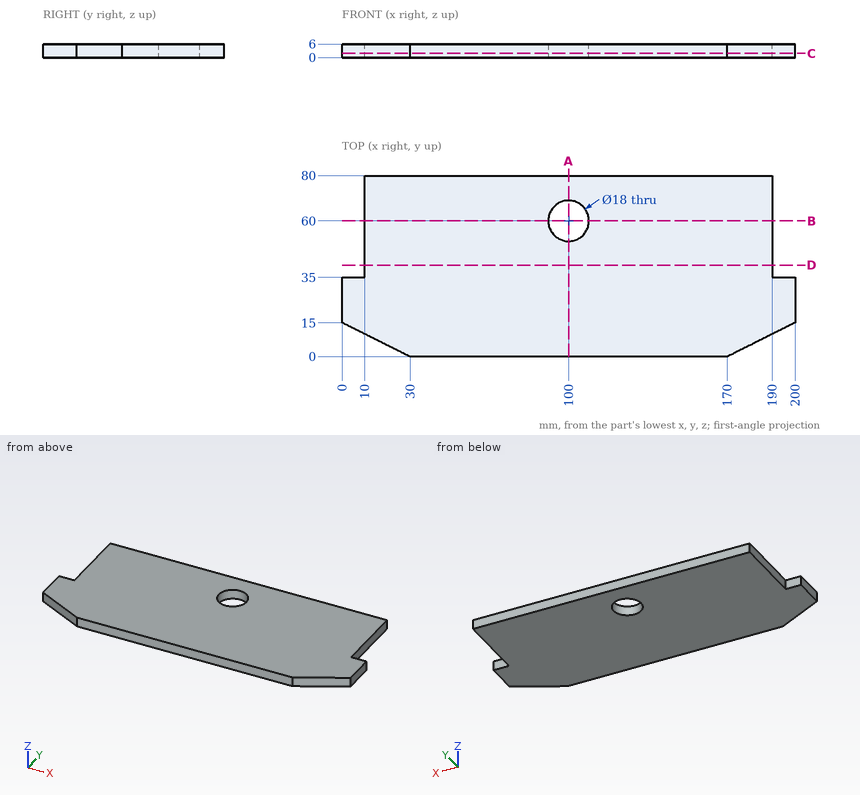
Source: three-view drawing plus pictorial views. Frame: mm from the lowest corner of the part. Give positions to 0.01 mm unless a question says otherwise; leave off trailing zeros. Loops run counter-clockwise (first coordinate to the right, second up) from the corner with the lowest first, then second, coordinate; pieces in that order, holes last.
1) Line query: L1, parallel to Y at x = 100, z = 3.3; L2, parallel to X at y = 38, z = 1.7; L3, parallel to X at y = 54.5, z = 5.4. Output: solid intervals per line, ascending.
A:
L1: y = 0 to 51, 69 to 80
L2: x = 10 to 190
L3: x = 10 to 92.88, 107.12 to 190
2) Section query D-D on y = 40.5. Return the cut outline in (x, z), and give its area (3 significant figures).
A:
outline: (10, 0) - (190, 0) - (190, 6) - (10, 6) - close
area: 1,080 mm2
3) Section query C-C on z = 1.9. Return the cut outline in (x, y).
A:
outline: (0, 15) - (30, 0) - (170, 0) - (200, 15) - (200, 35) - (190, 35) - (190, 80) - (10, 80) - (10, 35) - (0, 35) - close; hole circle Ø18 at (100, 60)
4) Section query B-B on y = 60. Return the cut outline in (x, z).
A:
outline: (10, 0) - (91, 0) - (91, 6) - (10, 6) - close; (109, 0) - (190, 0) - (190, 6) - (109, 6) - close
5) Contact query for flat-ended pins moving along their axis: pin 1 (1 mm diameter, centred on y = 11.5, z = 3, fed in from +X); pin 2 (1.8 mm diameter, centred on y = 62, z = 2.5, fed in from -X). Output: stop coordinate, or through.
A:
pin 1: stops at x = 194
pin 2: stops at x = 10
6) Section query A-A on x = 100. Return the cut outline in (y, z), and give its area (3 significant figures).
A:
outline: (0, 0) - (51, 0) - (51, 6) - (0, 6) - close; (69, 0) - (80, 0) - (80, 6) - (69, 6) - close
area: 372 mm2
